Input: part model. Units: mm. Frame: model coordinates. Face numbers are marked on the shaded views. Give positions to 0.01 mm unless a question says otherwise; leave off trailing zeros. Order: outer loops, then holes, each group sorted by start corner. A loop starts at its lowest first (then second) coordinate and runs counter-clockwise, first axis right, second up. Notation, with made-up numbers: (55.25, -12) - (74.25, -12) arc R29 ccw to (74.25, 22) - close; hole circle Ø8 at (17, 24.25). An arc over 180 degrees is marked (long way). Answer in a Markdown table with one row per item. Add a question column.
1. Contact query for flat-ended pins moving along their axis: pin 1 (6 mm diameter, centred on x = -27, y = 22.5, fed in from -Z); pin 2 (2 mm diameter, centred on y = -21, z = 24.5, fed in from +X); pin 3 (2 mm diameter, centred on x = 8.5, y = 4, fed in from -Z). Output: stop coordinate, or through.
2. Ray query, line 1 (X direction, y = -13, z = 46); line 2 (X direction, y = 28, z = 51); line 3 (Z direction, x = 0, y = -9.5). Return the intervals inside material, ascending. Write a range as [from, to].
3. Section query C-C on y = 1. Return loops of the section in (x, z).
4. Mould query, pull axis X, two halves, no side actions, for the marked faces 1, 2, 3 and 4. Classes: released by +X, released by -X, zero draft, split by the parting line, or undercut.
5. Section query D-D on x = -11.5. Return loops of the section in (y, z).
6. Section query B-B on y = -24. Return loops of the section in (x, z).
7. Section query A-A on z = 30. Return loops of the section in (x, y).
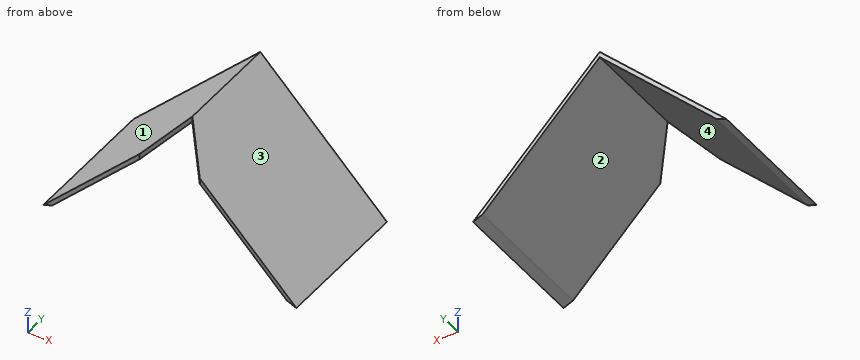
```python
from build123d import *

# Parameters (mm, degrees)
BOSS_EXTRUDE1_DEPTH     = 35
CUT_EXTRUDE3_DEPTH      = 96.198576189
CUT_EXTRUDE3_DEPTH_BACK = 96.198576189


with BuildPart() as part:
    # Sketch1 → Boss-Extrude1 (new, symmetric)
    with BuildSketch(Plane(origin=(0, 0, 0), x_dir=(1, 0, 0), z_dir=(0, 1, 0))):
        Polygon((-1.105e-06, -61.171572908), (-59.171572937, -2), (-64, 0), (-1.131e-06, -64.000000033), (64.000000066, 0), (59.171572879, -2), align=None)
    extrude(amount=BOSS_EXTRUDE1_DEPTH, both=True)

    # Sketch4 → Cut-Extrude3 (cut, two sides: drawn at the far end of the back side and taken through both)
    with BuildSketch(Plane.XY.offset(61.17).offset(-CUT_EXTRUDE3_DEPTH_BACK)):
        Polygon((-15.180001131, -35), (15.179998869, -35), (-1.131e-06, -17.5), align=None)
    extrude(amount=CUT_EXTRUDE3_DEPTH + CUT_EXTRUDE3_DEPTH_BACK, mode=Mode.SUBTRACT)


solid = part.part
```
Answer:
| question | item | result |
|---|---|---|
| 1 | pin 1 | stops at z = 31.17 |
| 1 | pin 2 | stops at x = 40.5 |
| 1 | pin 3 | stops at z = 51.67 |
| 2 | line 1 | x = [-18, -15.17], [15.17, 18] |
| 2 | line 2 | x = [-13, -10.17], [10.17, 13] |
| 2 | line 3 | z = [61.17, 64] |
| 3 | outline | (-64, 0) - (-59.17, 2) - (0, 61.17) - (59.17, 2) - (64, 0) - (0, 64) - close |
| 4 | face 1 | released by -X |
| 4 | face 2 | undercut |
| 4 | face 3 | released by +X |
| 4 | face 4 | undercut |
| 5 | outline | (-30.76, 49.67) - (35, 49.67) - (35, 52.5) - (-30.76, 52.5) - close |
| 6 | outline | (-64, 0) - (-59.17, 2) - (-5.64, 55.53) - (-5.64, 58.36) - close; (5.64, 55.53) - (59.17, 2) - (64, 0) - (5.64, 58.36) - close |
| 7 | outline | (-34, -35) - (-31.17, -35) - (-31.17, 35) - (-34, 35) - close; (31.17, -35) - (34, -35) - (34, 35) - (31.17, 35) - close |
